Design review of the part built by this model. Coordinates are the model's own, in mm. Face numbers are marked on the shaded views. A direction names the side the tool comes from. Give positions to 0.01 mm unless a question says otherwise; leave off trailing zeros. Write each loop counter-clockwise with the first axis right and the second up, starting at its lowest first coordinate (ties: lowest second). Pieces come first, ordered by that corner, then holes.
```python
from build123d import *

# Parameters (mm, degrees)
EXTRUDE_1_DEPTH      = 14
CUT_EXTRUDE_1_DEPTH  = 44
SKETCH_3_W           = 6.2
SKETCH_3_H           = 6.2
CUT_EXTRUDE_2_DEPTH  = 4
SKETCH_4_R           = 4
CUT_EXTRUDE_3_DEPTH  = 5
SKETCH_5_R           = 2.6
CUT_EXTRUDE_4_DEPTH  = 5
EXTRUDE_2_DEPTH      = 44
SKETCH_8_W           = 5
SKETCH_8_H           = 5
EXTRUDE_4_DEPTH      = 15
SKETCH_9_W           = 35
SKETCH_9_H           = 5
EXTRUDE_5_DEPTH      = 7
CUT_EXTRUDE_6_DEPTH  = 10
CUT_EXTRUDE_START    = -30
SKETCH_14_R          = 1.55
CUT_EXTRUDE_7_DEPTH  = 30
SKETCH_15_R          = 3
CUT_EXTRUDE_8_DEPTH  = 2
CUT_EXTRUDE_START_2  = -2
SKETCH_16_R          = 3
CUT_EXTRUDE_9_DEPTH  = 2
SKETCH_17_W          = 35
SKETCH_17_H          = 7
CUT_EXTRUDE_10_DEPTH = 10
SKETCH_18_W          = 35
SKETCH_18_H          = 7
CUT_EXTRUDE_11_DEPTH = 20


with BuildPart() as part:
    # 草图1 → 凸台-拉伸1 (new body)
    with BuildSketch(Plane.XY):
        Polygon((-15, 22), (-15, -22), (15, -22), (15, 22), (0, 22), align=None)
    extrude(amount=EXTRUDE_1_DEPTH)

    # 草图2 → 切除-拉伸1 (cut)
    with BuildSketch(Plane(origin=(0, 22, 0), x_dir=(1, 0, 0), z_dir=(0, 1, 0))):
        Polygon((-15, 0), (-15, -14), (-10, -4), (-3.1, -4), (-3.1, 0), align=None)
        Polygon((3.1, -4), (10, -4), (15, -14), (15, 0), (3.1, 0), align=None)
    extrude(amount=-CUT_EXTRUDE_1_DEPTH, mode=Mode.SUBTRACT)

    # 草图3 → 切除-拉伸2 (cut)
    with BuildSketch(Plane(origin=(0, 0, 0), x_dir=(-1, 0, 0), z_dir=(0, 0, -1))):
        Rectangle(SKETCH_3_W, SKETCH_3_H)
    extrude(amount=-CUT_EXTRUDE_2_DEPTH, mode=Mode.SUBTRACT)

    # 草图4 → 切除-拉伸3 (cut)
    with BuildSketch(Plane.XY.offset(14)):
        Circle(SKETCH_4_R)
    extrude(amount=-CUT_EXTRUDE_3_DEPTH, mode=Mode.SUBTRACT)

    # 草图5 → 切除-拉伸4 (cut)
    with BuildSketch(Plane.XY.offset(9)):
        Circle(SKETCH_5_R)
    extrude(amount=-CUT_EXTRUDE_4_DEPTH, mode=Mode.SUBTRACT)

    # 草图7 → 凸台-拉伸2 (add)
    with BuildSketch(Plane.XZ.offset(22)):
        Polygon((15, 14), (20, 14), (20, 9), (10, 4), (10, 14), align=None)
    extrude(amount=-EXTRUDE_2_DEPTH)

    # 草图8 → 凸台-拉伸4 (add)
    with BuildSketch(Plane.XY.offset(14)):
        with Locations((-12.5, -12.5)):
            Rectangle(SKETCH_8_W, SKETCH_8_H)
        Polygon((-10, -10), (-10, -15), (10, -15), (10, -10), (0, -10), align=None)
        Polygon((-10, 0), (-10, 10), (-15, 10), (-15, -10), (-10, -10), align=None)
        with Locations((-12.5, 12.5)):
            Rectangle(SKETCH_8_W, SKETCH_8_H)
        Polygon((-10, 15), (10, 15), (10, 10), (0, 10), (-10, 10), align=None)
        with Locations((12.5, 12.5)):
            Rectangle(SKETCH_8_W, SKETCH_8_H)
        Polygon((15, 10), (15, -10), (10, -10), (10, 0), (10, 10), align=None)
        with Locations((12.5, -12.5)):
            Rectangle(SKETCH_8_W, SKETCH_8_H)
        with Locations((17.5, -12.5)):
            Rectangle(SKETCH_8_W, SKETCH_8_H)
        with Locations((17.5, 12.5)):
            Rectangle(SKETCH_8_W, SKETCH_8_H)
    extrude(amount=EXTRUDE_4_DEPTH)

    # 草图9 → 凸台-拉伸5 (add)
    with BuildSketch(Plane(origin=(0, 15, 0), x_dir=(1, 0, 0), z_dir=(0, 1, 0))):
        with Locations((2.5, -26.5)):
            Rectangle(SKETCH_9_W, SKETCH_9_H)
    extrude(amount=EXTRUDE_5_DEPTH)

    # 草图13 → 切除-拉伸6 (cut)
    with BuildSketch(Plane(origin=(-10, 0, 0), x_dir=(0, 0, -1), z_dir=(1, 0, 0))):
        with BuildLine():
            ThreePointArc((-19.95, 0), (-20.806818927, 1.386362146), (-22.43, 1.24))
            Line((-22.43, 1.24), (-20.57, -1.24))
            ThreePointArc((-20.57, -1.24), (-20.113637854, -0.693181073), (-19.95, 0))
        make_face()
        with BuildLine():
            Line((-20.57, -1.24), (-22.43, 1.24))
            ThreePointArc((-22.43, 1.24), (-22.74, -0.93), (-20.57, -1.24))
        make_face()
    extrude(amount=-CUT_EXTRUDE_6_DEPTH, mode=Mode.SUBTRACT)

    # 草图14 → 切除-拉伸7 (cut)
    with BuildSketch(Plane.ZY.offset(15).offset(CUT_EXTRUDE_START)):
        with Locations(Location((21.5, 0, 0), (0, 0, 180))):
            Circle(SKETCH_14_R)
    extrude(amount=CUT_EXTRUDE_7_DEPTH, mode=Mode.SUBTRACT)

    # 草图15 → 切除-拉伸8 (cut)
    with BuildSketch(Plane(origin=(15, 0, 0), x_dir=(0, 0, -1), z_dir=(1, 0, 0))):
        with Locations((-21.5, 0)):
            Circle(SKETCH_15_R)
    extrude(amount=-CUT_EXTRUDE_8_DEPTH, mode=Mode.SUBTRACT)

    # 草图16 → 切除-拉伸9 (cut)
    with BuildSketch(Plane.ZY.offset(15).offset(CUT_EXTRUDE_START_2)):
        with Locations(Location((21.5, 0, 0), (0, 0, 180))):
            Circle(SKETCH_16_R)
    extrude(amount=CUT_EXTRUDE_9_DEPTH, mode=Mode.SUBTRACT)

    # 草图17 → 切除-拉伸10 (cut)
    with BuildSketch(Plane.XY.offset(29)):
        with Locations((2.5, 18.5)):
            Rectangle(SKETCH_17_W, SKETCH_17_H)
    extrude(amount=-CUT_EXTRUDE_10_DEPTH, mode=Mode.SUBTRACT)

    # 草图18 → 切除-拉伸11 (cut)
    with BuildSketch(Plane.XY.offset(14)):
        with Locations((2.5, 18.5)):
            Rectangle(SKETCH_18_W, SKETCH_18_H)
        with Locations((2.5, -18.5)):
            Rectangle(SKETCH_18_W, SKETCH_18_H)
    extrude(amount=-CUT_EXTRUDE_11_DEPTH, mode=Mode.SUBTRACT)


solid = part.part
```
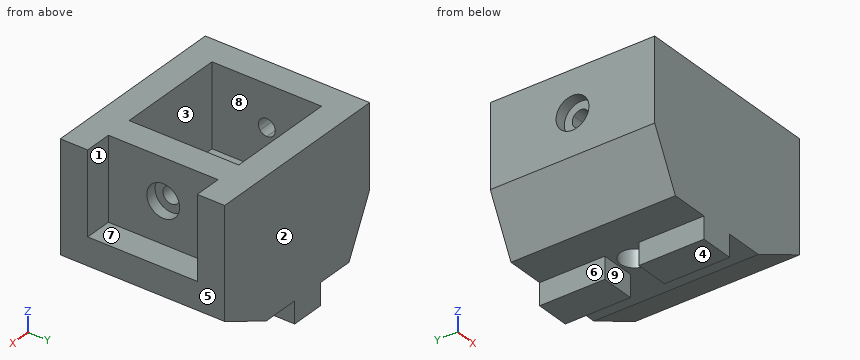
(1) Consider section A-A, the plane x = 0. Give the boundary of the cut face in (y, z), then the cut area to 3 significant figures.
Resolved:
outline: (-15, 0) - (-3.1, 0) - (-3.1, 4) - (-2.6, 4) - (-2.6, 9) - (-4, 9) - (-4, 14) - (-10, 14) - (-10, 29) - (-15, 29) - close; (2.6, 4) - (3.1, 4) - (3.1, 0) - (15, 0) - (15, 29) - (10, 29) - (10, 14) - (4, 14) - (4, 9) - (2.6, 9) - close
area: 479 mm2
(2) Consider section C-C, the plane z = 17. Give the boundary of the cut face in (x, y).
Resolved:
outline: (-15, -15) - (20, -15) - (20, -10) - (15, -10) - (15, 10) - (20, 10) - (20, 15) - (-15, 15) - close; hole (-10, -10) - (10, -10) - (10, 10) - (-10, 10) - close
(3) Consider section B-B, the plane z = 21.5. Give the boundary of the cut face in (x, y).
Resolved:
outline: (-15, -15) - (20, -15) - (20, -10) - (15, -10) - (15, -3) - (13, -3) - (13, -1.55) - (10, -1.55) - (10, -10) - (-10, -10) - (-10, -1.55) - (-13, -1.55) - (-13, -3) - (-15, -3) - close; (-15, 3) - (-13, 3) - (-13, 1.55) - (-10, 1.55) - (-10, 10) - (10, 10) - (10, 1.55) - (13, 1.55) - (13, 3) - (15, 3) - (15, 10) - (20, 10) - (20, 15) - (-15, 15) - close
(4) To check wall thickness, follow L1, parallel to Y at x = -13.8, z = 21.5; L2, parallel to Y at x = 0, z = 11.9; L3, parallel to X at y = -6, z = 17.75. State the ranges of each line that lie inside material, in increasing order.
Resolved:
L1: y = -15 to -3, 3 to 15
L2: y = -15 to -4, 4 to 15
L3: x = -15 to -10, 10 to 15
(5) Clearance check with flat-ended pins moving along their axes: P1, Ø3, axis at y = -11, z = 2, coming from the -X side; P2, Ø2, axis at y = -0.5, z = 24, coming from the +X side; P3, Ø3, axis at x = -5, y = 10, coming from the -Z side; P4, Ø4.5, axis at x = 0, y = 0, coming from the -Z side. State where each tip first meets the part, or that it passes through.
Resolved:
P1: stops at x = -3.1
P2: stops at x = 15
P3: stops at z = 4
P4: passes through
(6) Consider section D-D, the plane y = -2. Give the boundary of the cut face in (x, z).
Resolved:
outline: (-15, 14) - (-10, 4) - (-1.66, 4) - (-1.66, 9) - (-3.46, 9) - (-3.46, 14) - (-10, 14) - (-10, 29) - (-15, 29) - (-15, 23.74) - (-13, 23.74) - (-13, 19.26) - (-15, 19.26) - close; (1.66, 4) - (10, 4) - (20, 9) - (20, 14) - (15, 14) - (15, 19.26) - (13, 19.26) - (13, 23.74) - (15, 23.74) - (15, 29) - (10, 29) - (10, 14) - (3.46, 14) - (3.46, 9) - (1.66, 9) - close
(7) Tool access review of the marked faces 5, 6, 7, 8 and 9: name each direction out of +Z, -Z, +X, -X, +Y, -Y from which nothing blocks a thin tool from reaching the whole face with its end or side.
Resolved:
face 5: +Z, -Z, +X, +Y, -Y
face 6: -Z, -X, +Y, -Y
face 7: +Z, +X
face 8: +Z
face 9: -Z, +X, -X
(8) Mouldability with a two-part tool opening along Y and no side actions: class the marked faces 1, 2, 3 and 4 as pulls with the +Y half, pulls with the -Y half, needs draft (parallel to the pull), parting line crosses it, or undercut.
Resolved:
face 1: undercut
face 2: pulls with the +Y half
face 3: undercut
face 4: needs draft
